```python
from build123d import *

# Parameters (mm, degrees)
CYLINDER002_R           = 10.1
CYLINDER002_DEPTH       = 20
CYLINDER002_PITCH_ANGLE = 90
CYLINDER003_R           = 10.1
CYLINDER003_DEPTH       = 30
CYLINDER_R              = 12
CYLINDER_DEPTH          = 30
CYLINDER_PITCH_ANGLE    = 90
CYLINDER001_R           = 12
CYLINDER001_DEPTH       = 20


with BuildPart() as cylinder002:
    # Cylinder002 → Cylinder002 (new body)
    with BuildSketch(Plane.XY):
        Circle(CYLINDER002_R)
    extrude(amount=CYLINDER002_DEPTH)


with BuildPart() as cylinder002_1:
    # Cylinder002 pitch: moved
    add(cylinder002.part.rotate(Axis((0, 0, 0), (0, 1, 0)), CYLINDER002_PITCH_ANGLE))


with BuildPart() as cylinder002_2:
    # Cylinder002 placement: moved
    add(cylinder002_1.part.moved(Location((10, 0, 0))))


with BuildPart() as negative_fusion:
    # Cylinder003 → Cylinder003 (new body)
    with BuildSketch(Plane(origin=(0, -15, 0), x_dir=(0, 0, -1), z_dir=(0, 1, 0))):
        Circle(CYLINDER003_R)
    extrude(amount=CYLINDER003_DEPTH)

    # Fusion001: union Cylinder002
    add(cylinder002_2.part)


with BuildPart() as cylinder:
    # Cylinder → Cylinder (new body)
    with BuildSketch(Plane.XY):
        Circle(CYLINDER_R)
    extrude(amount=CYLINDER_DEPTH)


with BuildPart() as cylinder_1:
    # Cylinder pitch: moved
    add(cylinder.part.rotate(Axis((0, 0, 0), (0, 1, 0)), CYLINDER_PITCH_ANGLE))


with BuildPart() as cylinder_2:
    # Cylinder placement: moved
    add(cylinder_1.part)


with BuildPart() as cut:
    # Cylinder001 → Cylinder001 (new body)
    with BuildSketch(Plane(origin=(0, -10, 0), x_dir=(0, 0, -1), z_dir=(0, 1, 0))):
        Circle(CYLINDER001_R)
    extrude(amount=CYLINDER001_DEPTH)

    # Fusion: union Cylinder
    add(cylinder_2.part)

    # Cut: cut Negative Fusion
    add(negative_fusion.part, mode=Mode.SUBTRACT)


solid = cut.part
```
Design review of the part built by this model. Coordinates are the model's own, in mm. A direction names the side the tool comes from. Coordinates: 2 decimals unless noted, no trailing zeros. Order: outer loops, then holes, each group sorted by start corner. A loop starts at its lowest first (then second) coordinate and runs counter-clockwise, first axis right, second up. Notation, with made-up numbers: M 65.25,53 L 83.25,53 A16 ccw 83.25,70 Z; hole C -2,8.25 d2. An arc over 180 degrees is marked long. Answer as a JSON object with one key per item and string values. Group by question number.
1) Mouldability with a two-part tool opening along Y and no side actions: class faces 4 (the flat face through (10, 0, -5)), 5 (the cylindrical face through (18.12, 11.9, 1.56)), 6 (the flat face through (-10, -10, -3)) as pulls with the +Y half, pulls with the -Y half, needs draft (parallel to the pull), parting line crosses it, or undercut.
2) Add section D-D, the plane z = 4. Write out the cut boundary in (x, y), then the cut area to 3 significant figures.
3) For pin 1 (2 mm diameter, centred on x = 25, z = -5.5, fed in from +Y); pin 2 (2 mm diameter, centred on x = 2, y = -1, fed in from -Z); pin 3 (2.5 mm diameter, centred on y = 1, z = -5, fed in from +X); pin 4 (5 mm diameter, centred on x = 18, y = -4.5, fed in from +Z), all flat-tipped, find the tip position at first contact; note any pin that passes through.
4) Add section B-B, the plane x = 4.5. Write out the cut boundary in (y, z), then the cut area to 3 significant figures.
5) Wall thickness on L1, parallel to Z at x = 0, y = -7; L2, parallel to Z at x = -6, y = 5.5: over which ranges is each line inside the solid? List them lowest first.
6) Add section C-C, the plane y = 0. Write out the cut boundary in (x, z).
7) Tool access review of faces 1 (the cylindrical face through (-12, 0, 0)), 2 (the flat face through (30, -9, 5)), 3 (the cylindrical face through (19.86, 3.034, -9.634)): name each direction out of +Z, -Z, +X, -X, +Y, -Y from which nothing blocks a thin tool from reaching the whole face with its end or side.
8) Add section A-A, the plane z = 0. Write out the cut boundary in (x, y).
Computed values:
{
 "1": {"face 4": "undercut", "face 5": "parting line crosses it", "face 6": "pulls with the -Y half"},
 "2": {"outline": "M -11.31,-10 L -9.27,-10 L -9.27,10 L -11.31,10 Z; M 9.27,-11.31 L 30,-11.31 L 30,-9.27 L 10,-9.27 L 10,9.27 L 30,9.27 L 30,11.31 L 9.27,11.31 Z", "area": "139 mm^2"},
 "3": {"pin 1": "stops at y = 11.12", "pin 2": "stops at z = -12", "pin 3": "stops at x = 10", "pin 4": "stops at z = 11.83"},
 "4": {"outline": "M -10,-11.12 L -4.5,-11.12 A12 ccw 4.5,-11.12 L 10,-11.12 L 10,-9.04 L -10,-9.04 Z; M -10,9.04 L 10,9.04 L 10,11.12 L 4.5,11.12 A12 ccw -4.5,11.12 L -10,11.12 Z", "area": "93.9 mm^2"},
 "5": {"L1": "z = -12 to -10.1, 10.1 to 12", "L2": "z = -10.39 to -8.12, 8.12 to 10.39"},
 "6": {"outline": "M 0,-12 L 30,-12 L 30,-10.1 L 10,-10.1 L 10,-1.42 A10.1 cw long 10,1.42 L 10,10.1 L 30,10.1 L 30,12 L 0,12 A12 ccw Z"},
 "7": {"face 1": "none", "face 2": "+Z, -Z, +X, +Y, -Y", "face 3": "+X"},
 "8": {"outline": "M -12,-10 L -10.1,-10 L -10.1,10 L -12,10 Z; M 10.1,-12 L 30,-12 L 30,-10.1 L 10.1,-10.1 Z; M 10.1,10.1 L 30,10.1 L 30,12 L 10.1,12 Z"}
}
